from build123d import *

# Parameters (mm, degrees)
F0_W     = 200
F0_H     = 160
F1_DEPTH = 500
F2_SIZE2 = 75
F2_SIZE  = 100
F3_SIZE2 = 270
F3_SIZE  = 125


with BuildPart() as f1:
    # F0 (on Top) → F1 (new body)
    with BuildSketch(Plane.XY):
        with Locations((-100, -80)):
            Rectangle(F0_W, F0_H)
    extrude(amount=F1_DEPTH)

    # F2
    f2_edges = [f1.edges().sort_by_distance(p)[0] for p in [
        (-200, -80, 500),
    ]]
    f2_side = f1.faces().sort_by_distance((-100, -80, 500))[0]
    chamfer(f2_edges, length=F2_SIZE, length2=F2_SIZE2, reference=f2_side)

    # F3
    f3_edges = [f1.edges().sort_by_distance(p)[0] for p in [
        (-50, -160, 500),
    ]]
    f3_side = f1.faces().sort_by_distance((-50, -80, 500))[0]
    chamfer(f3_edges, length=F3_SIZE, length2=F3_SIZE2, reference=f3_side)


solid = f1.part
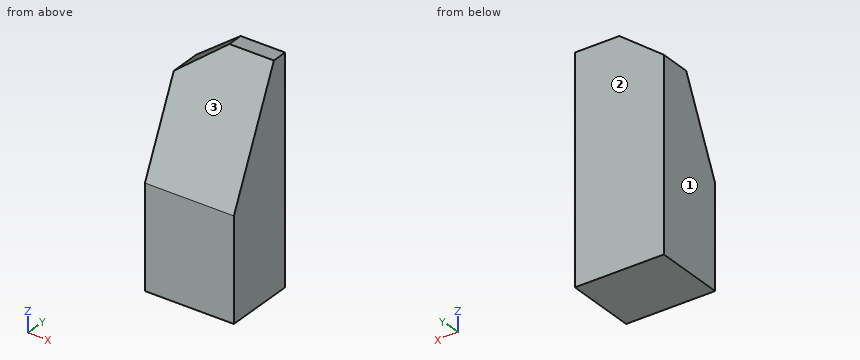
Model file for the job. Use its own axes, mm. Face numbers are marked on the shaded views. Give positions to 0.01 mm unless a question says otherwise; leave off trailing zeros. Write each loop counter-clockwise with the first axis right and the second up, starting at its lowest first coordinate (ties: lowest second). Pieces come first, ordered by that corner, then holes. Notation, with made-up numbers: M 68.25,29 L 114.25,29 A15 cw 114.25,53 Z; hole C 66,-31 d7. An arc over 180 degrees is marked long. One line per item, written item: value. Start each with the question number.
Q1. Saw through at B-B, the plane x = -41.5. Write the cut outline in (y, z), plus the area to 3 significant figures.
Q2. Saw through at A-A, the plane y = -61.5. Write the cut outline in (x, z).
Q3. Probe probe 1 along Z at (x, y) = (-45, -137.5); probe 2 along Y at (x, z) = (-84.5, 479.5); probe 3 along Z at (x, y) = (-102.5, -137). List the from-to ranges inside material, lowest first. Write a range as [from, to].
Q4. Saw through at C-C, the plane z = 461. Write the cut outline in (x, y), plus the area to 3 significant figures.
Q5. Two-plate mould, pull along Y, no slides. Class the marked faces 1, 2 and 3: +Y half, -Y half, draft (parallel to the pull), parting line (faces both ways), or undercut.
Q6. Saw through at D-D, the plane y = -125.5. Write the cut outline in (x, z), plus the area to 3 significant figures.
Q7. Drop a flat-ended pin along its axis: pin 1 Ø1.5 at (x, y) = (-167, -55) entering from +Z. Give the stop position or say it passes through.
Output values:
1. outline: M -160,0 L 0,0 L 0,500 L -35,500 L -160,230 Z
1. area: 63,100 mm²
2. outline: M -200,0 L 0,0 L 0,442.76 L -176.32,442.76 L -200,425 Z
3. probe 1: z = [0, 278.6]
3. probe 2: y = [-44.49, 0]
3. probe 3: z = [0, 279.68]
4. outline: M -152,-53.06 L 0,-53.06 L 0,0 L -152,0 Z
4. area: 8,060 mm²
5. face 1: draft
5. face 2: +Y half
5. face 3: -Y half
6. outline: M -200,0 L 0,0 L 0,304.52 L -200,304.52 Z
6. area: 60,900 mm²
7. pin 1: stops at z = 450.31
